Part model, mm, in its own coordinate system. A direction names the side the tool comes from. Give positions to 0.01 mm unless a question says otherwise; leave off trailing zeros. Write each loop counter-clockwise with the first axis right and the second up, starting at its lowest first coordinate (ties: lowest second). Pieces come first, ordered by that corner, then holes. Notation, with made-up numbers: M 88.25,-30 L 122.25,-30 A24 ccw 122.25,-20 Z; hole C 17.5,-15.75 d6. An arc over 180 degrees is marked long. Answer as CSV lines item,"result". Start each with the question number.
Item 1: Wall check: L1, parallel to Z at x = 5, y = 7.25; L2, parallel to Y at x = -30, z = 8.5; L3, parallel to X at y = 2.25, z = 15.5. Give the ranges that are in metal, low to high. Write a range as from..to.
Item 2: Pin check, flat tips, straight feed: pin 1 (2 mm diameter, centred on y = 7, z = 12.5, fed in from +X); pin 2 (2.5 mm diameter, centred on y = 1.5, z = 9, fed in from +X). Stop position of each tip, or through.
Item 3: Band-saw the part on B-B, the plane x = 0. List the corners of the cut face in (y, z).
Item 4: Band-saw the part on A-A, the plane z = 10.25. List the corners of the cut face in (x, y), then the cut area to 3 significant figures.
Item 5: 3-axis set-ups, long thin cutter, end or side, ignore diameter. For faces 1 (the cylindrical face through (134.77, 1.5, 8.87)), 2 (the flat face through (6, 0, 13)): which of +Z, -Z, +X, -X, +Y, -Y reach the whole face in a straight line?
Item 6: Band-saw the part on C-C, the plane y = 0. List the corners of the cut face in (x, z).
Item 7: Two-plate mould, pull along X, no slides. Class faces 3 (the cylindrical face through (-1.08, -4.88, 15.46)), 4 (the flat face through (51, 0, 0)), 5 (the cylindrical face through (-39, 0, 9)): +X half, -X half, draft (parallel to the pull), parting line (faces both ways), or undercut.
from build123d import *

# Parameters (mm, degrees)
SKETCH1_R           = 5
BOSS_EXTRUDE1_DEPTH = 18
SKETCH3_W           = 20
SKETCH3_H           = 8
CUT_EXTRUDE1_DEPTH  = 18


with BuildPart() as part:
    # Sketch1 → Boss-Extrude1 (new body)
    with BuildSketch(Plane.XY):
        with BuildLine():
            Line((-30, 9), (130, 9))
            ThreePointArc((130, 9), (139, 0), (130, -9))
            Line((130, -9), (-30, -9))
            ThreePointArc((-30, -9), (-39, 0), (-30, 9))
        make_face()
        Circle(SKETCH1_R, mode=Mode.SUBTRACT)
        with Locations((130, 0)):
            Circle(SKETCH1_R, mode=Mode.SUBTRACT)
        with Locations((-30, 0)):
            Circle(SKETCH1_R, mode=Mode.SUBTRACT)
    extrude(amount=BOSS_EXTRUDE1_DEPTH)

    # Sketch3 → Cut-Extrude1 (cut)
    with BuildSketch(Plane(origin=(0, 9, 0), x_dir=(1, 0, 0), z_dir=(0, 1, 0))):
        with Locations((1.222079484, -9)):
            Rectangle(SKETCH3_W, SKETCH3_H)
    extrude(amount=-CUT_EXTRUDE1_DEPTH, mode=Mode.SUBTRACT)


solid = part.part
Output:
1,L1,"0..5, 13..18"
1,L2,"-9..-5, 5..9"
1,L3,"-38.71..-34.47, -25.53..-4.47, 4.47..125.53, 134.47..138.71"
2,pin 1,"x = 136.71"
2,pin 2,"x = 139"
3,outline,"M -9,0 L -5,0 L -5,5 L -9,5 Z; M -9,13 L -5,13 L -5,18 L -9,18 Z; M 5,0 L 9,0 L 9,5 L 5,5 Z; M 5,13 L 9,13 L 9,18 L 5,18 Z"
4,outline,"M -30,-9 L -8.78,-9 L -8.78,9 L -30,9 A9 ccw Z; M 11.22,-9 L 130,-9 A9 ccw 130,9 L 11.22,9 Z; hole C -30,0 d10; hole C 130,0 d10"
4,area,"2,620 mm²"
5,face 1,"+Z, -Z"
5,face 2,"+Y, -Y"
6,outline,"M -39,0 L -35,0 L -35,18 L -39,18 Z; M -25,0 L -5,0 L -5,5 L -8.78,5 L -8.78,13 L -5,13 L -5,18 L -25,18 Z; M 5,0 L 125,0 L 125,18 L 5,18 L 5,13 L 11.22,13 L 11.22,5 L 5,5 Z; M 135,0 L 139,0 L 139,18 L 135,18 Z"
7,face 3,"undercut"
7,face 4,"draft"
7,face 5,"-X half"
